The listing builds one solid part. Answer for the finished solid, in the listing's coordinates (mm). A direction names the side the tool comes from. Round coordinates to 2 decimals unless told otherwise and drop trailing zeros. Loops run counter-clockwise (first coordinate to the right, second up) from the corner with the lowest first, then second, coordinate; pieces in that order, holes last. Notation, with made-up numbers: M -15,78 L 43,78 A11 cw 43,82 Z; hole C -22.75,-27 d2. An arc over 180 degrees is marked long. Put each result on its own line as item: value. Start each with the question number.
(1) A flat-ended cylindrical pin translates along its axis: P1, Ø1.6, axis at y = 0, z = 0, coming from the -X side. Find the tip coordinate at first contact, or state that the pin passes through.
(2) Determine the mould class of faces 4 (the face through (2.81, 1.14, 4.82)), 5 (the face through (0, -1, -1)), 6 (the face through (2.81, 4.938, 0.406)) for opening direction Y: released by +Y, released by -Y, zero draft, split by the parting line, or undercut.
(3) Which of the six approach directions +Z, -Z, +X, -X, +Y, -Y give full straight-line access (tool end or side, diameter ignored) to faces 1 (the face through (2.81, -1.14, 4.84)), 2 (the face through (2.81, -0.41, -4.95)), 3 (the face through (2.81, 3.765, -3.245))?
(4) Section A-A, the plane y = 0 is taken. Determine the outline of the cut face in (x, z).
(5) Section B-B, the plane x = 3.95 is taken. Count the separate pieces of the cut face and the enclosed holes in it, then the cut area to 3 significant figures.
(6) Straight lines are drawn through the part: line 1 (Z direction, x = 2.3, y = 4.5); line 2 (Y direction, x = 2.8, z = 3.75); line 3 (Z direction, x = 5.4, y = -4.75). For each, find the intervals that lie inside material, in ascending order.
(7) Section C-C, the plane z = 3 is taken. Determine the outline of the cut face in (x, y), then the cut area to 3 significant figures.
```python
from build123d import *

# Parameters (mm, degrees)
SKETCH_7_R      = 1
SKETCH_7_R_2    = 0.5
EXTRUDE_3_DEPTH = 5.7


with BuildPart() as part:
    # 草图7 → 凸台-拉伸3 (new body)
    with BuildSketch(Plane(origin=(0, 0, 0), x_dir=(0, 0, -1), z_dir=(1, 0, 0))):
        with BuildLine():
            ThreePointArc((-5.451006848, 0.732478218), (-4.945547363, 0.408928549), (-4.366855207, 0.249903181))
            ThreePointArc((-4.366855207, 0.249903181), (-4.374, 0), (-4.366855207, -0.249903181))
            ThreePointArc((-4.366855207, -0.249903181), (-4.945547363, -0.408928549), (-5.451006848, -0.732478218))
            ThreePointArc((-5.451006848, -0.732478218), (-5.432285873, -0.860389558), (-5.410563801, -0.987825571))
            ThreePointArc((-5.410563801, -0.987825571), (-4.829860918, -1.139344021), (-4.23035043, -1.111760422))
            ThreePointArc((-4.23035043, -1.111760422), (-4.159921202, -1.351640333), (-4.075901771, -1.58710452))
            ThreePointArc((-4.075901771, -1.58710452), (-4.577129176, -1.917172343), (-4.957867366, -2.381081934))
            ThreePointArc((-4.957867366, -2.381081934), (-4.900535883, -2.496947749), (-4.840497071, -2.61143411))
            ThreePointArc((-4.840497071, -2.61143411), (-4.241394034, -2.576089659), (-3.679749479, -2.364597169))
            ThreePointArc((-3.679749479, -2.364597169), (-3.538640333, -2.570972694), (-3.38597067, -2.76894901))
            ThreePointArc((-3.38597067, -2.76894901), (-3.760669693, -3.23774995), (-3.979417283, -3.796608762))
            ThreePointArc((-3.979417283, -3.796608762), (-3.889087297, -3.889087297), (-3.796608762, -3.979417283))
            ThreePointArc((-3.796608762, -3.979417283), (-3.23774995, -3.760669693), (-2.76894901, -3.38597067))
            ThreePointArc((-2.76894901, -3.38597067), (-2.570972694, -3.538640333), (-2.364597169, -3.679749479))
            ThreePointArc((-2.364597169, -3.679749479), (-2.576089659, -4.241394034), (-2.61143411, -4.840497071))
            ThreePointArc((-2.61143411, -4.840497071), (-2.496947749, -4.900535883), (-2.381081934, -4.957867366))
            ThreePointArc((-2.381081934, -4.957867366), (-1.917172343, -4.577129176), (-1.58710452, -4.075901771))
            ThreePointArc((-1.58710452, -4.075901771), (-1.351640333, -4.159921202), (-1.111760422, -4.23035043))
            ThreePointArc((-1.111760422, -4.23035043), (-1.139344021, -4.829860918), (-0.987825571, -5.410563801))
            ThreePointArc((-0.987825571, -5.410563801), (-0.860389558, -5.432285873), (-0.732478218, -5.451006848))
            ThreePointArc((-0.732478218, -5.451006848), (-0.408928549, -4.945547363), (-0.249903181, -4.366855207))
            ThreePointArc((-0.249903181, -4.366855207), (0, -4.374), (0.249903181, -4.366855207))
            ThreePointArc((0.249903181, -4.366855207), (0.408928549, -4.945547363), (0.732478218, -5.451006848))
            ThreePointArc((0.732478218, -5.451006848), (0.860389558, -5.432285873), (0.987825571, -5.410563801))
            ThreePointArc((0.987825571, -5.410563801), (1.139344021, -4.829860918), (1.111760422, -4.23035043))
            ThreePointArc((1.111760422, -4.23035043), (1.351640333, -4.159921202), (1.58710452, -4.075901771))
            ThreePointArc((1.58710452, -4.075901771), (1.917172343, -4.577129176), (2.381081934, -4.957867366))
            ThreePointArc((2.381081934, -4.957867366), (2.496947749, -4.900535883), (2.61143411, -4.840497071))
            ThreePointArc((2.61143411, -4.840497071), (2.576089659, -4.241394034), (2.364597169, -3.679749479))
            ThreePointArc((2.364597169, -3.679749479), (2.570972694, -3.538640333), (2.76894901, -3.38597067))
            ThreePointArc((2.76894901, -3.38597067), (3.23774995, -3.760669693), (3.796608762, -3.979417283))
            ThreePointArc((3.796608762, -3.979417283), (3.889087297, -3.889087297), (3.979417283, -3.796608762))
            ThreePointArc((3.979417283, -3.796608762), (3.760669693, -3.23774995), (3.38597067, -2.76894901))
            ThreePointArc((3.38597067, -2.76894901), (3.538640333, -2.570972694), (3.679749479, -2.364597169))
            ThreePointArc((3.679749479, -2.364597169), (4.241394034, -2.576089659), (4.840497071, -2.61143411))
            ThreePointArc((4.840497071, -2.61143411), (4.900535883, -2.496947749), (4.957867366, -2.381081934))
            ThreePointArc((4.957867366, -2.381081934), (4.577129176, -1.917172343), (4.075901771, -1.58710452))
            ThreePointArc((4.075901771, -1.58710452), (4.159921202, -1.351640333), (4.23035043, -1.111760422))
            ThreePointArc((4.23035043, -1.111760422), (4.829860918, -1.139344021), (5.410563801, -0.987825571))
            ThreePointArc((5.410563801, -0.987825571), (5.432285873, -0.860389558), (5.451006848, -0.732478218))
            ThreePointArc((5.451006848, -0.732478218), (4.945547363, -0.408928549), (4.366855207, -0.249903181))
            ThreePointArc((4.366855207, -0.249903181), (4.374, 0), (4.366855207, 0.249903181))
            ThreePointArc((4.366855207, 0.249903181), (4.945547363, 0.408928549), (5.451006848, 0.732478218))
            ThreePointArc((5.451006848, 0.732478218), (5.432285873, 0.860389558), (5.410563801, 0.987825571))
            ThreePointArc((5.410563801, 0.987825571), (4.829860918, 1.139344021), (4.23035043, 1.111760422))
            ThreePointArc((4.23035043, 1.111760422), (4.159921202, 1.351640333), (4.075901771, 1.58710452))
            ThreePointArc((4.075901771, 1.58710452), (4.577129176, 1.917172343), (4.957867366, 2.381081934))
            ThreePointArc((4.957867366, 2.381081934), (4.900535883, 2.496947749), (4.840497071, 2.61143411))
            ThreePointArc((4.840497071, 2.61143411), (4.241394034, 2.576089659), (3.679749479, 2.364597169))
            ThreePointArc((3.679749479, 2.364597169), (3.538640333, 2.570972694), (3.38597067, 2.76894901))
            ThreePointArc((3.38597067, 2.76894901), (3.760669693, 3.23774995), (3.979417283, 3.796608762))
            ThreePointArc((3.979417283, 3.796608762), (3.889087297, 3.889087297), (3.796608762, 3.979417283))
            ThreePointArc((3.796608762, 3.979417283), (3.23774995, 3.760669693), (2.76894901, 3.38597067))
            ThreePointArc((2.76894901, 3.38597067), (2.570972694, 3.538640333), (2.364597169, 3.679749479))
            ThreePointArc((2.364597169, 3.679749479), (2.576089659, 4.241394034), (2.61143411, 4.840497071))
            ThreePointArc((2.61143411, 4.840497071), (2.496947749, 4.900535883), (2.381081934, 4.957867366))
            ThreePointArc((2.381081934, 4.957867366), (1.917172343, 4.577129176), (1.58710452, 4.075901771))
            ThreePointArc((1.58710452, 4.075901771), (1.351640333, 4.159921202), (1.111760422, 4.23035043))
            ThreePointArc((1.111760422, 4.23035043), (1.139344021, 4.829860918), (0.987825571, 5.410563801))
            ThreePointArc((0.987825571, 5.410563801), (0.860389558, 5.432285873), (0.732478218, 5.451006848))
            ThreePointArc((0.732478218, 5.451006848), (0.408928549, 4.945547363), (0.249903181, 4.366855207))
            ThreePointArc((0.249903181, 4.366855207), (0, 4.374), (-0.249903181, 4.366855207))
            ThreePointArc((-0.249903181, 4.366855207), (-0.408928549, 4.945547363), (-0.732478218, 5.451006848))
            ThreePointArc((-0.732478218, 5.451006848), (-0.860389558, 5.432285873), (-0.987825571, 5.410563801))
            ThreePointArc((-0.987825571, 5.410563801), (-1.139344021, 4.829860918), (-1.111760422, 4.23035043))
            ThreePointArc((-1.111760422, 4.23035043), (-1.351640333, 4.159921202), (-1.58710452, 4.075901771))
            ThreePointArc((-1.58710452, 4.075901771), (-1.917172343, 4.577129176), (-2.381081934, 4.957867366))
            ThreePointArc((-2.381081934, 4.957867366), (-2.496947749, 4.900535883), (-2.61143411, 4.840497071))
            ThreePointArc((-2.61143411, 4.840497071), (-2.576089659, 4.241394034), (-2.364597169, 3.679749479))
            ThreePointArc((-2.364597169, 3.679749479), (-2.570972694, 3.538640333), (-2.76894901, 3.38597067))
            ThreePointArc((-2.76894901, 3.38597067), (-3.23774995, 3.760669693), (-3.796608762, 3.979417283))
            ThreePointArc((-3.796608762, 3.979417283), (-3.889087297, 3.889087297), (-3.979417283, 3.796608762))
            ThreePointArc((-3.979417283, 3.796608762), (-3.760669693, 3.23774995), (-3.38597067, 2.76894901))
            ThreePointArc((-3.38597067, 2.76894901), (-3.538640333, 2.570972694), (-3.679749479, 2.364597169))
            ThreePointArc((-3.679749479, 2.364597169), (-4.241394034, 2.576089659), (-4.840497071, 2.61143411))
            ThreePointArc((-4.840497071, 2.61143411), (-4.900535883, 2.496947749), (-4.957867366, 2.381081934))
            ThreePointArc((-4.957867366, 2.381081934), (-4.577129176, 1.917172343), (-4.075901771, 1.58710452))
            ThreePointArc((-4.075901771, 1.58710452), (-4.159921202, 1.351640333), (-4.23035043, 1.111760422))
            ThreePointArc((-4.23035043, 1.111760422), (-4.829860918, 1.139344021), (-5.410563801, 0.987825571))
            ThreePointArc((-5.410563801, 0.987825571), (-5.432285873, 0.860389558), (-5.451006848, 0.732478218))
        make_face()
        Circle(SKETCH_7_R, mode=Mode.SUBTRACT)
        with Locations((-0.605093134, 2.703102347)):
            Circle(SKETCH_7_R_2, mode=Mode.SUBTRACT)
    extrude(amount=EXTRUDE_3_DEPTH)


solid = part.part
```
Recorded:
1. P1: passes through
2. face 4: undercut
2. face 5: zero draft
2. face 6: released by +Y
3. face 1: +X, -X
3. face 2: -Z, +X, -X
3. face 3: +X, -X, +Y
4. outline: M 0,-4.37 L 5.7,-4.37 L 5.7,-1 L 0,-1 Z; M 0,1 L 5.7,1 L 5.7,4.37 L 0,4.37 Z
5. separate pieces: 1
5. enclosed holes: 2
5. area: 71.8 mm²
6. line 1: z = -2.61 to -1.85, -1.15 to -0.27, 0.27 to 1.15, 1.85 to 2.61
6. line 2: y = -3.97 to -3.22, -2.4 to 2.4, 3.22 to 3.97
6. line 3: z = -2.62 to -2.09, -1.15 to -0.33, 0.33 to 1.15, 2.09 to 2.62
7. outline: M 0,-3.6 L 5.7,-3.6 L 5.7,3.6 L 0,3.6 Z
7. area: 41.0 mm²
